Check sheet for the modelled part. Datum: model origin and axes. Units: mm. A direction names the side the tool comes from. Give positions to 0.01 mm unless a question says otherwise; leave off trailing zeros. Write each loop counter-clockwise with the first axis right and the second up, starting at its lowest first coordinate (ties: lowest second). Pieces come first, ordered by that corner, then holes. Notation, with made-up numbers: (74, 69) -> (117, 69) arc R17 cw to (117, 80) -> close; hole circle Ø6 at (7, -19). An arc over 180 degrees is marked (long way). Use a Markdown table: item, result. Add a question column.
1. Release check for a two-part mould opening along X. For faces 5 (the flat face through (-1, 12.7, 10)), 6 (the cylindrical face through (-22.37, 0.95, 12.88)), 7 (the cylindrical face through (-39.628, 0.178, 14.149)) record: released by +X, released by -X, zero draft, split by the parting line, or undercut.
2. Scan lines: probe 1 along X at (y, z) = (0, 20.25) (3 decimals); probe 2 along Y at (x, z) = (-25.4, 10.5) (3 decimals); probe 3 along X at (y, z) = (-10.5, 20). Record each from-to range of solid material in increasing order. Write a range as [from, to].
3. Gauge pin test, flat ends, axial feed: P1, Ø1.9, axis at y = 6, z = 22, coming from the -X side; P2, Ø5, axis at x = 13, y = 7, coming from the -Z side; P3, Ø4.5, axis at x = 1, y = -1.5, coming from the +Z side; P4, Ø5.5, axis at x = -50.8, y = 0, coming from the -Z side (3 decimals). Record the tip position at first contact, or that the pin passes through.
4. Cross-section at C-C (y = 4.5). Enter the section's corners in (x, z), then the cut area to 3 significant figures.
5. Cross-section at B-B (x = 50.8). Enter the section's corners in (y, z) (3 decimals), then the cut area to 3 significant figures.
6. Cross-section at D-D (z = 8.5). Enter the section's corners in (x, y) (3 decimals).
7. Set-up check for faces 1 (the cylindrical face through (28.43, 0.95, 12.88)), 2 (the flat face through (56, 0, 12.7)), 3 (the cylindrical face through (-11.251, -0.178, 14.228)), 4 (the flat face through (-55, 0, 12.7)): record each of +Z, -Z, +X, -X, +Y, -Y from which the full face is reachable in a straight line by a thin tool's end or side.
8. Cross-section at A-A (z = 22). Enter the section's corners in (x, y) (3 decimals).
from build123d import *

# Parameters (mm, degrees)
F1_DEPTH      = 12.7
F1_DEPTH_BACK = 12.7
F2_R          = 3.175
F3_DEPTH      = 12.701
F3_DEPTH_BACK = 12.701
F4_R          = 5.08
F5_SIZE       = 1.27


with BuildPart() as f1:
    # F0 (on Front) → F1 (new body, two sides)
    with BuildSketch(Plane.XZ) as f1_sk:
        Polygon((-63.5, 12.7), (-63.5, 0), (63.5, 0), (63.5, 12.7), (38.1, 12.7), (38.1, 25.4), (12.7, 25.4), (12.7, 12.7), (-12.7, 12.7), (-12.7, 25.4), (-38.1, 25.4), (-38.1, 12.7), align=None)
    extrude(amount=F1_DEPTH)
    extrude(f1_sk.sketch, amount=-F1_DEPTH_BACK)

    # F2 (on face) → F3 (cut, two sides)
    with BuildSketch(Plane.XY.offset(12.7)) as f3_sk:
        with Locations((-50.8, 0)):
            Circle(F2_R)
        with Locations((50.8, 0)):
            Circle(F2_R)
        with Locations((-25.4, 0)):
            Circle(F2_R)
        with Locations((25.4, 0)):
            Circle(F2_R)
    extrude(amount=-F3_DEPTH, mode=Mode.SUBTRACT)
    extrude(f3_sk.sketch, amount=F3_DEPTH_BACK, mode=Mode.SUBTRACT)

    # F4
    f4_edges = [f1.edges().sort_by_distance(p)[0] for p in [
        (-38.1, 0, 12.7),
        (12.7, 0, 12.7),
        (-12.7, 0, 12.7),
        (38.1, 0, 12.7),
    ]]
    fillet(f4_edges, radius=F4_R)

    # F5
    f5_edges = [f1.edges().sort_by_distance(p)[0] for p in [
        (-25.4, -12.7, 25.4),
        (-12.7, 0, 25.4),
        (-25.4, 12.7, 25.4),
        (-38.1, 0, 25.4),
        (12.7, 0, 25.4),
        (25.4, 12.7, 25.4),
        (38.1, 0, 25.4),
        (25.4, -12.7, 25.4),
    ]]
    chamfer(f5_edges, length=F5_SIZE)


solid = f1.part
Worked answers:
| question | item | result |
|---|---|---|
| 1 | face 5 | zero draft |
| 1 | face 6 | undercut |
| 1 | face 7 | released by -X |
| 2 | probe 1 | x = [-38.1, -28.575], [-22.225, -12.7], [12.7, 22.225], [28.575, 38.1] |
| 2 | probe 2 | y = [-12.7, -3.175], [3.175, 12.7] |
| 2 | probe 3 | x = [-38.1, -12.7], [12.7, 38.1] |
| 3 | P1 | stops at x = -38.1 |
| 3 | P2 | stops at z = 0 |
| 3 | P3 | stops at z = 12.7 |
| 3 | P4 | passes through |
| 4 | outline | (-63.5, 0) -> (63.5, 0) -> (63.5, 12.7) -> (43.18, 12.7) arc R5.08 cw to (38.1, 17.78) -> (38.1, 24.13) -> (36.83, 25.4) -> (13.97, 25.4) -> (12.7, 24.13) -> (12.7, 17.78) arc R5.08 cw to (7.62, 12.7) -> (-7.62, 12.7) arc R5.08 cw to (-12.7, 17.78) -> (-12.7, 24.13) -> (-13.97, 25.4) -> (-36.83, 25.4) -> (-38.1, 24.13) -> (-38.1, 17.78) arc R5.08 cw to (-43.18, 12.7) -> (-63.5, 12.7) -> close |
| 4 | area | 2,280 mm² |
| 5 | outline | (-12.7, 0) -> (-3.175, 0) -> (-3.175, 12.7) -> (-12.7, 12.7) -> close; (3.175, 0) -> (12.7, 0) -> (12.7, 12.7) -> (3.175, 12.7) -> close |
| 5 | area | 242 mm² |
| 6 | outline | (-63.5, -12.7) -> (63.5, -12.7) -> (63.5, 12.7) -> (-63.5, 12.7) -> close; hole circle Ø6.35 at (-50.8, 0); hole circle Ø6.35 at (-25.4, 0); hole circle Ø6.35 at (25.4, 0); hole circle Ø6.35 at (50.8, 0) |
| 7 | face 1 | +Z, -Z |
| 7 | face 2 | +Z, +X, +Y, -Y |
| 7 | face 3 | +Z, +Y, -Y |
| 7 | face 4 | +Z, -X, +Y, -Y |
| 8 | outline | (-38.1, -12.7) -> (-12.7, -12.7) -> (-12.7, 12.7) -> (-38.1, 12.7) -> close; (12.7, -12.7) -> (38.1, -12.7) -> (38.1, 12.7) -> (12.7, 12.7) -> close; hole circle Ø6.35 at (-25.4, 0); hole circle Ø6.35 at (25.4, 0) |
